Can you work these out from the model? Positions are in its coordinate system, mm. A direction names the side the tool comes from. Coordinates: 2 decimals unless noted, no trailing zeros. Order: outer loops, then holes, each group sorted by start corner. A loop starts at its lowest first (then second) coordinate and runs counter-clockwise, first axis right, second up. Notation, with made-up numbers: (-22, 33.5) -> (35, 33.5) arc R18 cw to (35, 46.5) -> close; hole circle Ø3 at (38, 0.5). An arc over 180 degrees is marked (long way). Answer as CSV lines item,"result".
from build123d import *

# Parameters (mm, degrees)
SKETCH3_W           = 12.7
SKETCH3_H           = 35
SKETCH3_W_2         = 40
SKETCH3_H_2         = 12.7
BOSS_EXTRUDE1_DEPTH = 12.7
SKETCH4_W           = 40
SKETCH4_H           = 12.7
CUT_EXTRUDE1_DEPTH  = 12.7
SKETCH5_W           = 40
SKETCH5_H           = 12.7
SKETCH5_W_2         = 70
SKETCH5_H_2         = 40
CUT_EXTRUDE2_DEPTH  = 12.7


with BuildPart() as part:
    # Sketch3 → Boss-Extrude1 (new body)
    with BuildSketch(Plane.XY):
        Polygon((127.7, 60), (-127.7, 60), (-127.7, -25), (-127.7, -60), (-20, -60), (20, -60), (127.7, -60), (127.7, -25), align=None)
        with Locations((-134.05, -42.5)):
            Rectangle(SKETCH3_W, SKETCH3_H)
        with Locations((134.05, -42.5)):
            Rectangle(SKETCH3_W, SKETCH3_H)
        with Locations((0, -66.35)):
            Rectangle(SKETCH3_W_2, SKETCH3_H_2)
    extrude(amount=BOSS_EXTRUDE1_DEPTH)

    # Sketch4 → Cut-Extrude1 (cut)
    with BuildSketch(Plane.XY.offset(12.7)):
        with Locations((0, 53.65)):
            Rectangle(SKETCH4_W, SKETCH4_H)
    extrude(amount=-CUT_EXTRUDE1_DEPTH, mode=Mode.SUBTRACT)

    # Sketch5 → Cut-Extrude2 (cut)
    with BuildSketch(Plane.XY.offset(12.7)):
        with Locations((-75.7, 53.65)):
            Rectangle(SKETCH5_W, SKETCH5_H)
        with Locations((75.7, 53.65)):
            Rectangle(SKETCH5_W, SKETCH5_H)
        with Locations((-60.7, 7.3)):
            Rectangle(SKETCH5_W_2, SKETCH5_H_2)
        with Locations((60.7, 7.3)):
            Rectangle(SKETCH5_W_2, SKETCH5_H_2)
    extrude(amount=-CUT_EXTRUDE2_DEPTH, mode=Mode.SUBTRACT)


solid = part.part
Q1. Which directions (+Z, -Z, +X, -X, +Y, -Y) give clear straight access to the entire face, cutting with the end or side of a thin tool? Please do faces 4 (the flat face through (60, 27.3, 6)), 5 (the flat face through (127.7, 17, 6)), 6 (the flat face through (55.7, 54, 6)).
Solution:
face 4,"+Z, -Z"
face 5,"+Z, -Z, +X, +Y"
face 6,"+Z, -Z, +Y"
Q2. If I drill on line 1 (X direction, y = -4, z = 11.75); line 2 (Y direction, x = -55.5, z = 6); line 3 (Y direction, x = -79.5, z = 9.5), over which ranges is the centre line in solid material (lowest first)?
Solution:
line 1,"-127.7 to -95.7, -25.7 to 25.7, 95.7 to 127.7"
line 2,"-60 to -12.7, 27.3 to 60"
line 3,"-60 to -12.7, 27.3 to 47.3"
Q3. For P1, Ø6, axis at x = -64.5, z = 5.5, coming from the -Y side; P2, Ø5, axis at x = -67, z = 2.5, coming from the +Y side; P3, Ø1.5, axis at x = 34.5, y = -36, coming from the -Z side; P4, Ø4, axis at y = -2, z = 5.5, coming from the -X side, each with a flat end and sliding along its axis, tell me the tip position at first contact or that it passes through.
Solution:
P1,"y = -60"
P2,"y = 47.3"
P3,"z = 0"
P4,"x = -127.7"
Q4. Imagine slicing it at D-D (x = -108). List the corners of the cut face in (y, z) for me, and give its area (3 significant figures).
Solution:
outline,"(-60, 0) -> (60, 0) -> (60, 12.7) -> (-60, 12.7) -> close"
area,"1,520 mm2"
Q5. We'd pull the mould along Y, two halves only. Please class faces 1 (the flat face through (-61, -12.7, 6)), 2 (the flat face through (0, 47.3, 6)), 3 (the flat face through (-81, -60, 6)): pulls with the +Y half, pulls with the -Y half, needs draft (parallel to the pull), parting line crosses it, or undercut.
Solution:
face 1,"undercut"
face 2,"pulls with the +Y half"
face 3,"pulls with the -Y half"
Q6. Imagine slicing it at A-A (y = -6.5). List the corners of the cut face in (x, z) for me, and give its area (3 significant figures).
Solution:
outline,"(-127.7, 0) -> (-95.7, 0) -> (-95.7, 12.7) -> (-127.7, 12.7) -> close; (-25.7, 0) -> (25.7, 0) -> (25.7, 12.7) -> (-25.7, 12.7) -> close; (95.7, 0) -> (127.7, 0) -> (127.7, 12.7) -> (95.7, 12.7) -> close"
area,"1,470 mm2"
Q7. Imagine slicing it at C-C (z = 10). Give the number of separate pieces and of enclosed holes in the cut face, and give its area (3 significant figures).
Solution:
separate pieces,"1"
enclosed holes,"2"
area,"24,900 mm2"
Q8. Imagine slicing it at B-B (x = -70.5). List the corners of the cut face in (y, z) for me.
Solution:
outline,"(-60, 0) -> (-12.7, 0) -> (-12.7, 12.7) -> (-60, 12.7) -> close; (27.3, 0) -> (47.3, 0) -> (47.3, 12.7) -> (27.3, 12.7) -> close"
